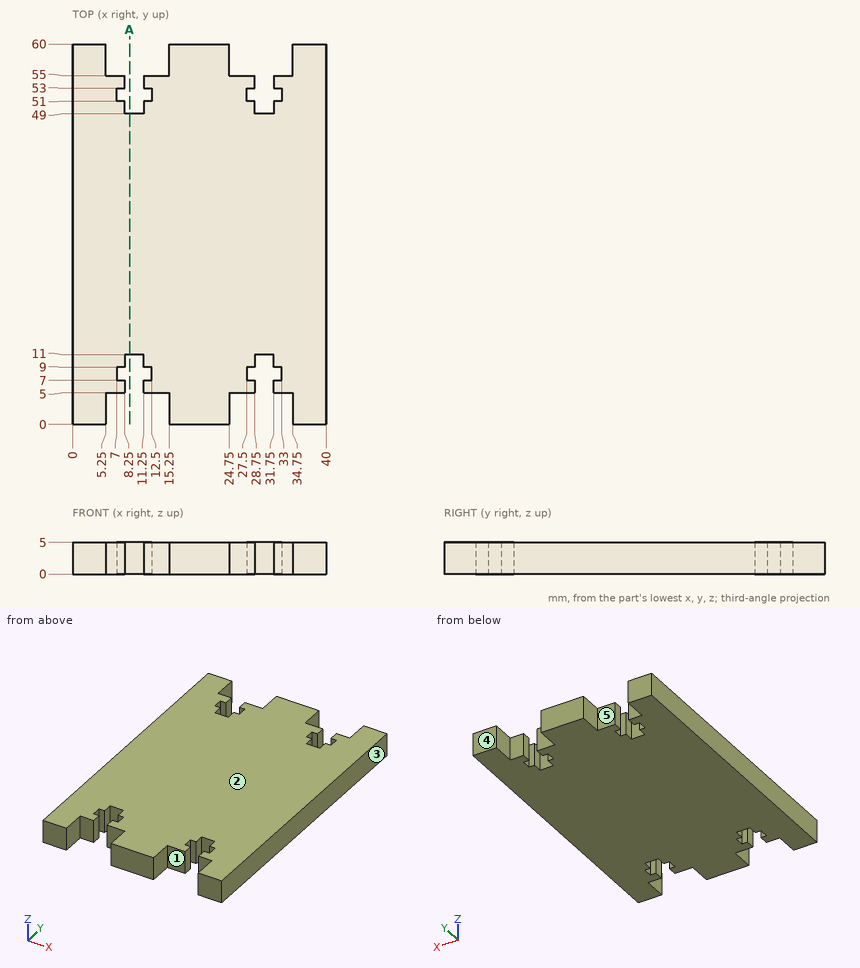
Study the drawing (mm; zero at the part's minimum x, y, z) and answer. A direction names the side the tool comes from. Coordinates: 2 decimals unless noted, no trailing zeros. Order: outer loops, then holes, each group sorted by start corner. A loop starts at its lowest first (then second) coordinate and runs counter-clockwise, first axis right, second up. Notation, with made-up numbers: M 21,29.5 L 70,29.5 A9 ccw 70,33.5 Z; hole C 38.25,-30 d8. An arc over 180 degrees is marked long. Answer as a JSON object with one key per item and string values. Group by question number.
1. Section A-A on x = 9 is taken. Write down the section's boundary in (y, z).
2. A tool of negligible diameter and unlimited length cuts with its end or side. For the marked faces 4 and 5, from which of +Z, -Z, +X, -X, +Y, -Y can it reach the whole face along a straight path? Write none if from no direction.
3. Straight lines are drawn through the part: line 1 (Y direction, x = 32.5, z = 4.7); line 2 (X direction, y = 52.5, z = 3.2); line 3 (X direction, y = 5.5, z = 1.1). For each, find the intervals that lie inside material, in ascending order.
4. Flat-ended cylindrical pins translate along their axes: P1, Ø0.9, axis at x = 31, z = 3, coming from the +Y side; P2, Ø0.6, axis at x = 32.5, z = 2.5, coming from the +Y side; P3, Ø1.2, axis at x = 26.5, z = 3.5, coming from the -Y side. Find the tip coordinate at first contact, or state that the pin passes through.
5. Determine the mould class of the marked faces 1, 2 and 3 for opening direction X: released by +X, released by -X, zero draft, split by the parting line, or undercut.
Values follow:
{
 "1": {"outline": "M 11,0 L 49,0 L 49,5 L 11,5 Z"},
 "2": {"face 4": "+Z, -Z, +X, -X, +Y", "face 5": "+Z, -Z, +Y"},
 "3": {"line 1": "5 to 7, 9 to 51, 53 to 55", "line 2": "0 to 7, 12.5 to 27.5, 33 to 40", "line 3": "0 to 8.25, 11.25 to 28.75, 31.75 to 40"},
 "4": {"P1": "y = 49", "P2": "y = 55", "P3": "y = 5"},
 "5": {"face 1": "undercut", "face 2": "zero draft", "face 3": "released by +X"}
}
